```python
from build123d import *

# Parameters (mm, degrees)
SKETCH1_W           = 133.5
SKETCH1_H           = 75
SKETCH1_R           = 1.725
BOSS_EXTRUDE1_DEPTH = 8
SKETCH2_W           = 107
SKETCH2_H           = 75
BOSS_EXTRUDE2_DEPTH = 29.65
CUT_EXTRUDE1_DEPTH  = 32.65
SKETCH4_W           = 2
SKETCH4_H           = 6.5
BOSS_EXTRUDE3_DEPTH = 32.65
FILLET1_R           = 5
FILLET4_R           = 1


with BuildPart() as part:
    # Sketch1 → Boss-Extrude1 (new body)
    with BuildSketch(Plane.XY):
        Rectangle(SKETCH1_W, SKETCH1_H)
        with Locations((-58.35, 0)):
            Circle(SKETCH1_R, mode=Mode.SUBTRACT)
        with Locations((58.35, 0)):
            Circle(SKETCH1_R, mode=Mode.SUBTRACT)
    extrude(amount=BOSS_EXTRUDE1_DEPTH)

    # Sketch2 → Boss-Extrude2 (add)
    with BuildSketch(Plane(origin=(0, 0, 0), x_dir=(-1, 0, 0), z_dir=(0, 0, -1))):
        Rectangle(SKETCH2_W, SKETCH2_H)
    extrude(amount=BOSS_EXTRUDE2_DEPTH)

    # Sketch3 → Cut-Extrude1 (cut)
    with BuildSketch(Plane.XY.offset(8)):
        Polygon((-38.95, 33.85), (-38.95, 27.35), (-40.95, 27.35), (-40.95, 33.85), (-50.35, 33.85), (-50.35, 1.75), (50.25, 1.75), (50.25, 33.85), (40.85, 33.85), (40.85, 27.35), (38.85, 27.35), (38.85, 33.85), (29.45, 33.85), (29.45, 27.35), (27.45, 27.35), (27.45, 33.85), (18.05, 33.85), (18.05, 27.35), (16.05, 27.35), (16.05, 33.85), (6.65, 33.85), (6.65, 27.35), (4.65, 27.35), (4.65, 33.85), (-4.75, 33.85), (-4.75, 27.35), (-6.75, 27.35), (-6.75, 33.85), (-16.15, 33.85), (-16.15, 27.35), (-18.15, 27.35), (-18.15, 33.85), (-27.55, 33.85), (-27.55, 27.35), (-29.55, 27.35), (-29.55, 33.85), align=None)
    cut_extrude1 = extrude(amount=-CUT_EXTRUDE1_DEPTH, mode=Mode.SUBTRACT)

    # Mirror1: Cut-Extrude1 across plane
    add(cut_extrude1.mirror(Plane.ZX), mode=Mode.SUBTRACT)

    # Sketch4 → Boss-Extrude3 (add)
    with BuildSketch(Plane.XY.offset(8)):
        with Locations((-39.95, 5)):
            Rectangle(SKETCH4_W, SKETCH4_H)
        with Locations((-28.55, 5)):
            Rectangle(SKETCH4_W, SKETCH4_H)
        with Locations((-17.15, 5)):
            Rectangle(SKETCH4_W, SKETCH4_H)
        with Locations((-5.75, 5)):
            Rectangle(SKETCH4_W, SKETCH4_H)
        with Locations((5.65, 5)):
            Rectangle(SKETCH4_W, SKETCH4_H)
        with Locations((17.05, 5)):
            Rectangle(SKETCH4_W, SKETCH4_H)
        with Locations((28.45, 5)):
            Rectangle(SKETCH4_W, SKETCH4_H)
        with Locations((39.85, 5)):
            Rectangle(SKETCH4_W, SKETCH4_H)
    boss_extrude3 = extrude(amount=-BOSS_EXTRUDE3_DEPTH)

    # Mirror2: Boss-Extrude3 across plane
    add(boss_extrude3.mirror(Plane.ZX))

    # Fillet1
    fillet1_edges = [part.edges().sort_by_distance(p)[0] for p in [
        (-66.75, 37.5, 4),
        (66.75, 37.5, 4),
        (66.75, -37.5, 4),
        (-66.75, -37.5, 4),
    ]]
    fillet(fillet1_edges, radius=FILLET1_R)

    # Fillet4
    fillet4_edges = [part.edges().sort_by_distance(p)[0] for p in [
        (53.5, 37.5, -14.825),
        (53.5, -37.5, -14.825),
        (-53.5, -37.5, -14.825),
        (-53.5, 37.5, -14.825),
        (53.5, 0, -29.65),
        (0, -37.5, -29.65),
        (-53.5, 0, -29.65),
        (0, 37.5, -29.65),
    ]]
    fillet(fillet4_edges, radius=FILLET4_R)


solid = part.part
```
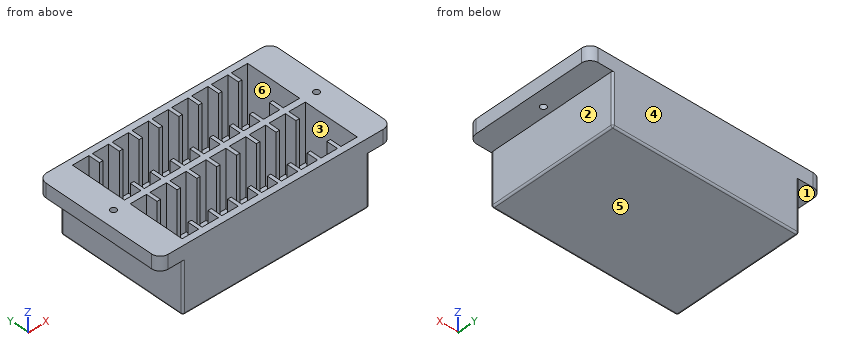
Could you check a few things on this model? Use its own coordinates, in mm. Face numbers are marked on the shaded views. A direction names the side the tool comes from. Round coordinates to 2 decimals unless told otherwise and drop trailing zeros. Order: outer loops, then holes, each group sorted by start corner. A loop starts at its lowest first (then second) coordinate and runs counter-clockwise, first axis right, second up. Notation, with made-up numbers: M 7.5,66.25 L 46.5,66.25 A21 cw 46.5,103.25 Z; hole C 41.5,22.25 d7. An arc over 180 degrees is marked long. One line per question, with ' | ' between items. Start each with the question number.
(1) For the marked faces 1, 2 and 3, which set-ups out of +Z, -Z, +X, -X, +Y, -Y let a thin tool reach every point of the face, with its end or its side?
(2) Suppose I cut it at A-A on y = 0. List the corners of the cut face in (x, z) for me (3 decimals), then the cut area to 3 significant figures.
(3) Suppose I cut it at C-C on y = -24.5. List the corners of the cut face in (x, z) for me, then the cut area to 3 significant figures.
(4) Suppose I cut it at D-D on x = -58.35. List the corners of the cut face in (y, z) for me (3 decimals), then the cut area to 3 significant figures.
(5) Please list where these lines run through material, in increasing order: line 1 along Y through (x, z) = (44, 6); line 2 along X through (y, z) = (8.5, -14); line 3 along Y through (x, z) = (-58.35, 6) (3 decimals).
(6) For P1, Ø2, axis at y = 3.5, z = -2.5, coming from the -X side; P2, Ø2, axis at y = 6.5, z = -12.5, coming from the +X side, each with a flat end and sliding along its axis, tell me the tip position at first contact or that it passes through.
(7) Thinking about a two-plate mould opening in Y: for the marked faces 4, 5 and 6, which applies, +Y half, -Y half, draft (parallel to the pull), parting line (faces both ways), or undercut?
(8) Suppose I cut it at B-B on x = 11. List the corners of the cut face in (y, z) for me.
Geometry results:
1) face 1: -Z, -X, +Y, -Y | face 2: -Z, +X, +Y, -Y | face 3: +Z
2) outline: M -66.75,0 L -60.075,0 L -60.075,8 L -66.75,8 Z; M -56.625,0 L -53.5,0 L -53.5,-28.65 A1 ccw -52.5,-29.65 L 52.5,-29.65 A1 ccw 53.5,-28.65 L 53.5,0 L 56.625,0 L 56.625,8 L -56.625,8 Z; M 60.075,0 L 66.75,0 L 66.75,8 L 60.075,8 Z | area: 4,180 mm²
3) outline: M -66.75,0 L -53.5,0 L -53.5,-28.65 A1 ccw -52.5,-29.65 L 52.5,-29.65 A1 ccw 53.5,-28.65 L 53.5,0 L 66.75,0 L 66.75,8 L 50.25,8 L 50.25,-24.65 L -50.35,-24.65 L -50.35,8 L -66.75,8 Z | area: 956 mm²
4) outline: M -37.5,0 L -1.725,0 L -1.725,8 L -37.5,8 Z; M 1.725,0 L 37.5,0 L 37.5,8 L 1.725,8 Z | area: 572 mm²
5) line 1: -37.5 to -33.85, -1.75 to 1.75, 33.85 to 37.5 | line 2: -53.5 to -50.35, 50.25 to 53.5 | line 3: -37.5 to -1.725, 1.725 to 37.5
6) P1: x = -53.5 | P2: x = 53.5
7) face 4: +Y half | face 5: draft | face 6: undercut
8) outline: M -37.5,-28.65 A1 ccw -36.5,-29.65 L 36.5,-29.65 A1 ccw 37.5,-28.65 L 37.5,8 L 33.85,8 L 33.85,-24.65 L 1.75,-24.65 L 1.75,8 L -1.75,8 L -1.75,-24.65 L -33.85,-24.65 L -33.85,8 L -37.5,8 Z
